from build123d import *

# Parameters (mm, degrees)
SKETCH1_R                 = 1.45
BOSS_EXTRUDE1_DEPTH       = 3
SKETCH4_W                 = 3.5
SKETCH4_H                 = 12
BOSS_EXTRUDE3_DEPTH       = 10.5
SKETCH5_W                 = 2
SKETCH5_H                 = 12
BOSS_EXTRUDE4_DEPTH       = 1.1
SKETCH6_W                 = 0.2
SKETCH6_H                 = 3
BOSS_EXTRUDE5_DEPTH       = 0.5
CHAMFER1_SIZE             = 10.5
F_3_0MM_DOWEL_HOLE1_D     = 2.9
F_3_0MM_DOWEL_HOLE1_DEPTH = 13.5
SKETCH10_R                = 1.45
BOSS_EXTRUDE6_DEPTH       = 3
CUT_EXTRUDE1_START        = -2
SKETCH11_R                = 1.45
CUT_EXTRUDE1_DEPTH        = 2


with BuildPart() as part:
    # Sketch1 → Boss-Extrude1 (new body)
    with BuildSketch(Plane(origin=(0, 0, 0), x_dir=(1, 0, 0), z_dir=(0, 1, 0))):
        with BuildLine():
            Line((-49, 6), (49, 6))
            ThreePointArc((49, 6), (55, 0), (49, -6))
            Line((49, -6), (-49, -6))
            ThreePointArc((-49, -6), (-55, 0), (-49, 6))
        make_face()
        with Locations(Location((-51.5, 0, 0), (0, 0, 270))):
            Circle(SKETCH1_R, mode=Mode.SUBTRACT)
        with Locations(Location((51.5, 0, 0), (0, 0, 270))):
            Circle(SKETCH1_R, mode=Mode.SUBTRACT)
    extrude(amount=BOSS_EXTRUDE1_DEPTH)

    # Sketch4 → Boss-Extrude3 (add)
    with BuildSketch(Plane.XZ):
        with Locations((-21.690023983, 0)):
            Rectangle(SKETCH4_W, SKETCH4_H)
        with Locations((21.690023983, 0)):
            Rectangle(SKETCH4_W, SKETCH4_H)
    extrude(amount=BOSS_EXTRUDE3_DEPTH)

    # Sketch5 → Boss-Extrude4 (add)
    with BuildSketch(Plane.XZ):
        with Locations((5, 0)):
            Rectangle(SKETCH5_W, SKETCH5_H)
        Rectangle(SKETCH5_W, SKETCH5_H)
        with Locations((10, 0)):
            Rectangle(SKETCH5_W, SKETCH5_H)
        with Locations((-5, 0)):
            Rectangle(SKETCH5_W, SKETCH5_H)
        with Locations((-10, 0)):
            Rectangle(SKETCH5_W, SKETCH5_H)
    extrude(amount=BOSS_EXTRUDE4_DEPTH)

    # Sketch6 → Boss-Extrude5 (add)
    with BuildSketch(Plane.XY.offset(6)):
        with Locations((48.9, 1.5)):
            Rectangle(SKETCH6_W, SKETCH6_H)
        with Locations((-48.9, 1.5)):
            Rectangle(SKETCH6_W, SKETCH6_H)
    extrude(amount=BOSS_EXTRUDE5_DEPTH)

    # Chamfer1
    chamfer1_edges = [part.edges().sort_by_distance(p)[0] for p in [
        (23.440023983, 0, 0),
        (-23.440023983, 0, 0),
    ]]
    chamfer(chamfer1_edges, length=CHAMFER1_SIZE - 0.0001)  # a hair under: the kernel refuses the full size

    # Ø3.0mm Dowel Hole1
    with Locations(Plane(origin=(0, 3, 0), x_dir=(1, 0, 0), z_dir=(0, 1, 0))):
        with Locations((-51.5, 0), (51.5, 0)):
            Hole(F_3_0MM_DOWEL_HOLE1_D / 2, depth=F_3_0MM_DOWEL_HOLE1_DEPTH)

    # Sketch10 → Boss-Extrude6 (add)
    # profile 1 of 2: a face of its own
    with BuildSketch(Plane(origin=(0, 3, 0), x_dir=(1, 0, 0), z_dir=(0, 1, 0))):
        with BuildLine():
            Line((-48.8, -6), (-27.05, -6))
            Line((-27.05, -6), (-27.05, 6))
            Line((-27.05, 6), (-49, 6))
            ThreePointArc((-49, 6), (-55, 0), (-49, -6))
            Line((-49, -6), (-49, -6.5))
            Line((-49, -6.5), (-48.8, -6.5))
            Line((-48.8, -6.5), (-48.8, -6))
        make_face()
        with Locations(Location((-51.5, 0, 0), (0, 0, 270.000000001))):
            Circle(SKETCH10_R, mode=Mode.SUBTRACT)
    # profile 2 of 2: a face of its own
    with BuildSketch(Plane(origin=(0, 3, 0), x_dir=(1, 0, 0), z_dir=(0, 1, 0))):
        with BuildLine():
            Line((27.05, 6), (27.05, -6))
            Line((27.05, -6), (48.8, -6))
            Line((48.8, -6), (48.8, -6.5))
            Line((48.8, -6.5), (49, -6.5))
            Line((49, -6.5), (49, -6))
            ThreePointArc((49, -6), (55, 0), (49, 6))
            Line((49, 6), (27.05, 6))
        make_face()
        with Locations(Location((51.5, 0, 0), (0, 0, 270))):
            Circle(SKETCH10_R, mode=Mode.SUBTRACT)
    extrude(amount=BOSS_EXTRUDE6_DEPTH)

    # Sketch11 → Cut-Extrude1 (cut)
    # profile 1 of 2: a face of its own
    with BuildSketch(Plane(origin=(0, 6, 0), x_dir=(1, 0, 0), z_dir=(0, 1, 0)).offset(CUT_EXTRUDE1_START)):
        Polygon((53.08771324, 2.75), (54.675426481, 0), (53.08771324, -2.75), (49.91228676, -2.75), (48.324573519, 0), (49.91228676, 2.75), align=None)
    # profile 2 of 2: a face of its own
    with BuildSketch(Plane(origin=(0, 6, 0), x_dir=(1, 0, 0), z_dir=(0, 1, 0)).offset(CUT_EXTRUDE1_START)):
        Polygon((-48.324573519, 0), (-49.91228676, 2.75), (-53.08771324, 2.75), (-54.675426481, 0), (-53.08771324, -2.75), (-49.91228676, -2.75), align=None)
        with Locations(Location((-51.5, 0, 0), (0, 0, 270.000000001))):
            Circle(SKETCH11_R, mode=Mode.SUBTRACT)
    extrude(amount=CUT_EXTRUDE1_DEPTH, mode=Mode.SUBTRACT)


solid = part.part
Geometry check sheet. Reference: the model listing, model coordinates, mm. A direction names the side the tool comes from. Round coordinates to 2 decimals unless told otherwise and drop trailing zeros. Order: outer loops, then holes, each group sorted by start corner. A loop starts at its lowest first (then second) coordinate and runs counter-clockwise, first axis right, second up. Notation, with made-up numbers: (62, 65) -> (116, 65) arc R28 ccw to (116, 90) -> close; hole circle Ø2 at (20, -27). An arc over 180 degrees is marked (long way). Use one line per item in the form item = value.
1. Cross-section at C-C, the plane y = -5.25. Enter the section's corners in (x, z), plus the area to 3 significant figures.
Working result:
outline = (-28.69, -6) -> (-19.94, -6) -> (-19.94, 6) -> (-28.69, 6) -> close; (19.94, -6) -> (28.69, -6) -> (28.69, 6) -> (19.94, 6) -> close
area = 210 mm^2
2. Mould release check, pull along Z, two halves, no side actions. Record for faces 1 (the face through (49.13, 4.986, 1.394)), 2 (the face through (-2, 0, 0)), 3 (the face through (-0.7, -0.5, 6)): pulls with the +Z half, pulls with the -Z half, needs draft (parallel to the pull), parting line crosses it, or undercut.
Working result:
face_1 = undercut
face_2 = needs draft
face_3 = pulls with the +Z half
3. Scan lines: line 1 along X through (y, z) = (1.35, 0); line 2 along Y through (x, z) = (-9.5, 2.75); line 3 along Y through (x, z) = (34.5, 3.5). Record each from-to range of solid material in increasing order. Write a range as from..to.
Working result:
line_1 = -55..-52.95, -50.05..50.05, 52.95..55
line_2 = -1.1..3
line_3 = 0..6
4. Cross-section at A-A, the plane y = 1.5. Enter the section's corners in (x, z), plus the area to 3 significant figures.
Working result:
outline = (-49, -6) -> (49, -6) arc R6 ccw to (49, 6) -> (49, 6.5) -> (48.8, 6.5) -> (48.8, 6) -> (-48.8, 6) -> (-48.8, 6.5) -> (-49, 6.5) -> (-49, 6) arc R6 ccw to start; hole circle Ø2.9 at (-51.5, 0); hole circle Ø2.9 at (51.5, 0)
area = 1,280 mm^2
5. Set-up check for faces 4 (the face through (-15, 0, 0)), 5 (the face through (-50, 4, -1)), 6 (the face through (-38, 6, 0)): record each of +Z, -Z, +X, -X, +Y, -Y from which the full face is reachable in a straight line by a thin tool's end or side.
Working result:
face_4 = +Z, -Z, -Y
face_5 = +Y
face_6 = +Z, -Z, +X, -X, +Y
6. Go/stop test with flat-tipped pins: pin 1 (0.9 mm diameter, centred on y = -0.5, z = -1.5, fed in from +X); pin 2 (5 mm diameter, centred on x = -19.5, z = 0.5, fed in from +Y); pin 3 (1.5 mm diameter, centred on y = 1.5, z = -2, fed in from +X). Record where each tip stops, or that it passes through.
Working result:
pin_1 = 33.89
pin_2 = 3
pin_3 = 54.87
7. Cross-section at B-B, the plane x = -51.5. Enter the section's corners in (y, z), plus the area to 3 significant figures.
Working result:
outline = (0, -5.45) -> (6, -5.45) -> (6, -2.75) -> (4, -2.75) -> (4, -1.45) -> (0, -1.45) -> close; (0, 1.45) -> (4, 1.45) -> (4, 2.75) -> (6, 2.75) -> (6, 5.45) -> (0, 5.45) -> close
area = 42.9 mm^2
